Can you work these out from the model? Positions are in its coordinate system, mm. Face numbers are marked on the shaded views. A direction names the side the tool comes from. Round coordinates to 2 decimals unless told otherwise and drop trailing zeros. Loops run counter-clockwise (first coordinate to the right, second up) from the corner with the lowest first, then second, coordinate; pieces in that order, holes last. Notation, with made-up numbers: M 47,55 L 105,55 A28 cw 105,86 Z; hole C -35.5,77 d6. An arc over 180 degrees is marked long. Use a Markdown table: item, result. Add a question column.
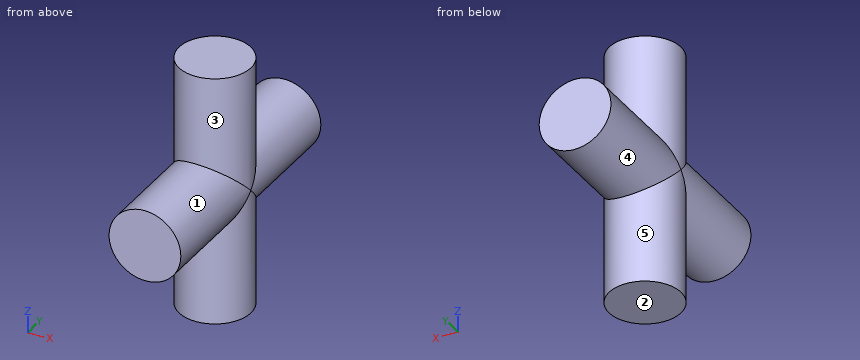
```python
from build123d import *

# Parameters (mm, degrees)
SKETCH1_R                = 3.175
BOSS_EXTRUDE1_DEPTH      = 11.1125
BOSS_EXTRUDE1_DEPTH_BACK = 11.1125
SKETCH2_R                = 3.175
BOSS_EXTRUDE2_DEPTH      = 11.1125
BOSS_EXTRUDE2_DEPTH_BACK = 11.1125


with BuildPart() as part:
    # Sketch1 → Boss-Extrude1 (new body, two sides)
    with BuildSketch(Plane.XY) as boss_extrude1_sk:
        Circle(SKETCH1_R)
    extrude(amount=BOSS_EXTRUDE1_DEPTH)
    extrude(boss_extrude1_sk.sketch, amount=-BOSS_EXTRUDE1_DEPTH_BACK)

    # Sketch2 → Boss-Extrude2 (add, two sides)
    with BuildSketch(Plane(origin=(0, 0, 0), x_dir=(1, 0, 0), z_dir=(0, 1, 0))) as boss_extrude2_sk:
        Circle(SKETCH2_R)
    extrude(amount=BOSS_EXTRUDE2_DEPTH)
    extrude(boss_extrude2_sk.sketch, amount=-BOSS_EXTRUDE2_DEPTH_BACK)


solid = part.part
```
(1) If I drill on probe 1 along Y at (x, z) = (0, 6.25) (3 decimals); probe 2 along Y at (x, z) = (1.75, 4.5), over which ranges is the centre line in solid material (lowest first)? Write a range as [from, to].
(2) Suppose I cut it at C-C on y = 7.75. List the corners of the cut face in (x, z) for me (3 decimals).
(3) On a 3-axis mill with a long thin cutter (end or side, diameter ignored), from which of +Z, -Z, +X, -X, +Y, -Y can I reach the whole of each face in a straight line? I mean the marked faces 1, 2, 3, 4 and 5. Say none if no direction works.
(4) I'm going to push flat-ended pins straight in: pin 1 (12 mm diameter, centred on y = -3, z = -6.5, fed in from +X) (3 decimals); pin 2 (1 mm diameter, centred on x = -2.5, z = -6, fed in from +Y); pin 3 (1.5 mm diameter, centred on x = 1, z = -8.5, fed in from -Y); pin 4 (4 mm diameter, centred on y = -4, z = -8.5, fed in from +X). Where does each tip first touch, or does it pass through?
(5) Suppose I cut it at A-A on x = 0. List the corners of the cut face in (y, z) for me (1 decimal).
Results below:
| question | item | result |
|---|---|---|
| 1 | probe 1 | y = [-3.175, 3.175] |
| 1 | probe 2 | y = [-2.65, 2.65] |
| 2 | outline | C 0,0 d6.35 |
| 3 | face 1 | -Y |
| 3 | face 2 | -Z, +X, -X, +Y, -Y |
| 3 | face 3 | +Z |
| 3 | face 4 | +Y |
| 3 | face 5 | -Z |
| 4 | pin 1 | stops at x = 3.175 |
| 4 | pin 2 | stops at y = 2.47 |
| 4 | pin 3 | stops at y = -3.17 |
| 4 | pin 4 | stops at x = 2.47 |
| 5 | outline | M -11.1,-3.2 L -3.2,-3.2 L -3.2,-11.1 L 3.2,-11.1 L 3.2,-3.2 L 11.1,-3.2 L 11.1,3.2 L 3.2,3.2 L 3.2,11.1 L -3.2,11.1 L -3.2,3.2 L -11.1,3.2 Z |
